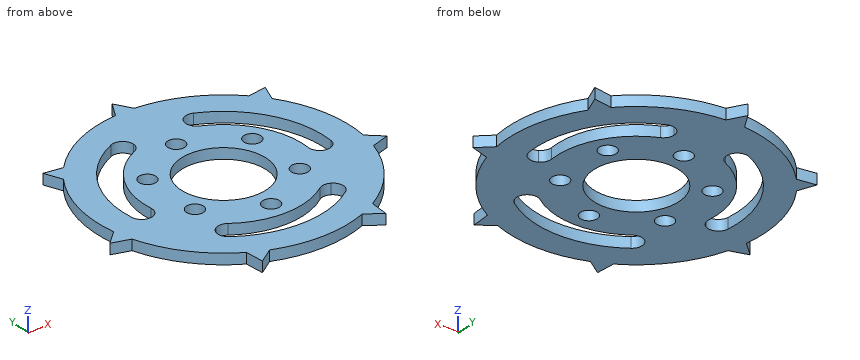
Autodesk Fusion 360 part; units mm, degrees
sketch "Sketch1" plane through (0, 0, 0) normal (0, 0, 1) x (1, 0, 0)
  circle A0 centre (0, 0) radius 24
  circle A1 centre (0, 0) radius 11.5
  line L0 (0, 0) -> (0, 11.5)
  line L1 (0, 0) -> (-9.9593, 5.75)
  line L2 (0, 0) -> (9.9593, 5.75)
  line L3 (0, 0) -> (9.9593, -5.75)
  line L4 (0, 0) -> (0, -11.5)
  line L5 (0, 0) -> (-9.9593, -5.75)
  circle A2 centre (0, 11.5) radius 1.6
  circle A3 centre (9.9593, 5.75) radius 1.6
  circle A4 centre (9.9593, -5.75) radius 1.6
  circle A5 centre (0, -11.5) radius 1.6
  circle A6 centre (-9.9593, -5.75) radius 1.6
  circle A7 centre (-9.9593, 5.75) radius 1.6
  line L6 (0, 11.5) -> (-5, 11.5)
  line L7 (0, 11.5) -> (5, 11.5)
  line L8 (9.9593, -5.75) -> (7.4593, -10.0801)
  line L9 (9.9593, -5.75) -> (12.4593, -1.4199)
  line L10 (-9.9593, -5.75) -> (-7.4593, -10.0801)
  line L11 (-9.9593, -5.75) -> (-12.4593, -1.4199)
  circle A8 centre (0, 0) radius 19
  line L12 (-5, 11.5) -> (-5, 10.3562)
  line L13 (5, 11.5) -> (5, 10.3562)
  line L14 (12.4593, -1.4199) -> (11.4687, -0.848)
  line L15 (7.4593, -10.0801) -> (6.4687, -9.5082)
  line L16 (-7.4593, -10.0801) -> (-6.4687, -9.5082)
  line L17 (-12.4593, -1.4199) -> (-11.4687, -0.848)
  line L18 (-12.4593, -1.4199) -> (-18.3745, -4.835)
  line L19 (-7.4593, -10.0801) -> (-13.3745, -13.4953)
  line L20 (7.4593, -10.0801) -> (13.3745, -13.4953)
  line L21 (12.4593, -1.4199) -> (18.3745, -4.835)
  line L22 (5, 11.5) -> (5, 18.3303)
  line L23 (-5, 11.5) -> (-5, 18.3303)
  circle A9 centre (0, 0) radius 8
  circle A10 centre (0, 0) radius 15
  line L24 (0, 24) -> (-15.4269, 18.3851)
  line L25 (-15.4269, 18.3851) -> (-23.6354, 4.1676)
  line L26 (-23.6354, 4.1676) -> (-20.7846, -12)
  line L27 (-20.7846, -12) -> (-8.2085, -22.5526)
  line L28 (-8.2085, -22.5526) -> (8.2085, -22.5526)
  line L29 (8.2085, -22.5526) -> (20.7846, -12)
  line L30 (20.7846, -12) -> (23.6354, 4.1676)
  line L31 (23.6354, 4.1676) -> (15.4269, 18.3851)
  line L32 (15.4269, 18.3851) -> (0, 24)
  line L33 (0, 24) -> (0.2615, 26.9886)
  line L34 (0, 24) -> (3, 24) construction
  line L35 (0.2615, 26.9886) -> (-1.883, 23.926)
  line L36 (0.2615, 26.9886) -> (4.0002, 26.9886) construction
  dimension "d1" = 48
  dimension "d2" = 23
  dimension "d3" = 3.2
  dimension "d4" = 3.2
  dimension "d5" = 3.2
  dimension "d6" = 3.2
  dimension "d7" = 3.2
  dimension "d8" = 3.2
  dimension "d9" = 5
  dimension "d10" = 5
  dimension "d11" = 5
  dimension "d12" = 5
  dimension "d13" = 5
  dimension "d14" = 38
  dimension "d15" = 16
  dimension "d16" = 30
  dimension "d17" = 85
  dimension "d18" = 3
  dimension "d19" = 125
extrude "Extrude1" add sketch "Sketch1" along normal blind 2 contours A0 L30 | A0 L31 | L24 L25 L26 L27 L28 L29 L30 L31 L32 | A0 L29 | A0 L32 | A0 L28 | A0 L24 | A0 L27 | A0 L25 | A0 L26 | A1 L2 L3 A3 A4 A9 | A1 A4 L9 L14 | A1 A3 L13 L14 L21 L22 A10 | A4 L8 L9 L20 L21 A10 | A1 L3 L4 A4 A5 A9 | A8 L20 L21 A10 | A1 L0 L2 A2 A3 A9 | A1 A4 L8 L15 | A1 A5 L15 L16 L19 L20 A10 | A1 L4 L5 A5 A6 A9 | A6 L10 L11 L18 L19 A10 | A8 L18 L19 A10 | A8 L22 L23 A10 | A2 L6 L7 L22 L23 A10 | A1 A2 L7 L13 | A1 L0 L1 A2 A7 A9 | A1 L1 L5 A6 A7 A9 | A1 A6 L10 L16 | A1 A7 L12 L17 L18 L23 A10 | A1 A6 L11 L17 | A1 A2 L6 L12
fillet "Fillet1" radius 2 12 edges at (5, 18.3303, 1) (5, 14.1421, 1) (14.7474, -2.7409, 1) (18.3745, -4.835, 1) (13.3745, -13.4953, 1) (9.7474, -11.4012, 1) (-9.7474, -11.4012, 1) (-13.3745, -13.4953, 1) (-18.3745, -4.835, 1) (-14.7474, -2.7409, 1) (-5, 14.1421, 1) (-5, 18.3303, 1)
sketch "Sketch2" plane through (0, 0, 2) normal (0, 0, 1) x (-1, 0, 0)
  circle A0 centre (9.9593, 5.75) radius 1.6
  circle A1 centre (0, 0) radius 8
  circle A2 centre (0, -11.5) radius 1.6
  arc A3 (8.7498, 12.1837) -> (11.083, 15.4326) centre (9.9164, 13.8081) ccw
  arc A4 (8.7498, 12.1837) -> (-8.7498, 12.1837) centre (0, 0) ccw
  arc A5 (-11.083, 15.4326) -> (-8.7498, 12.1837) centre (-9.9164, 13.8081) ccw
  arc A6 (11.083, 15.4326) -> (-11.083, 15.4326) centre (0, 0) ccw
  circle A7 centre (9.9593, -5.75) radius 1.6
  arc A8 (6.1765, -13.6694) -> (7.8235, -17.3145) centre (7, -15.4919) ccw
  arc A9 (6.1765, -13.6694) -> (14.9262, 1.4857) centre (0, 0) ccw
  arc A10 (18.9066, 1.8819) -> (14.9262, 1.4857) centre (16.9164, 1.6838) ccw
  arc A11 (7.8235, -17.3145) -> (18.9066, 1.8819) centre (0, 0) ccw
  arc A12 (-18.9066, 1.8819) -> (-7.8235, -17.3145) centre (0, 0) ccw
  arc A13 (-14.9262, 1.4857) -> (-18.9066, 1.8819) centre (-16.9164, 1.6838) ccw
  arc A14 (-14.9262, 1.4857) -> (-6.1765, -13.6694) centre (0, 0) ccw
  arc A15 (-7.8235, -17.3145) -> (-6.1765, -13.6694) centre (-7, -15.4919) ccw
  circle A16 centre (-9.9593, -5.75) radius 1.6
  circle A17 centre (0, 11.5) radius 1.6
  circle A18 centre (-9.9593, 5.75) radius 1.6
  circle A19 centre (0, 0) radius 24
  line L0 (0, -8) -> (0, -13.1)
  line L1 (0, -24) -> (3.0935, -24) construction
  line L2 (0, -24) -> (0, -27)
  line L3 (0, -24) -> (3.0102, -24) construction
  line L4 (0, -27) -> (1.7698, -23.9347)
  line L5 (0, -27) -> (-1.7698, -23.9347)
  arc A20 (0, -27) -> (0, -27) centre (0, 0) ccw
  arc A21 (-1.7698, -23.9347) -> (1.7698, -23.9347) centre (0, 0) ccw
  line L6 (21.1095, -16.8342) -> (19.8163, -13.5393)
  line L7 (21.1095, -16.8342) -> (17.6094, -16.3067)
  arc A22 (17.6094, -16.3067) -> (19.8163, -13.5393) centre (0, 0) ccw
  line L8 (26.3231, 6.0081) -> (22.9408, 7.0514)
  line L9 (26.3231, 6.0081) -> (23.7284, 3.6006)
  arc A23 (23.7284, 3.6006) -> (22.9408, 7.0514) centre (0, 0) ccw
  line L10 (11.7149, 24.3262) -> (8.7903, 22.3323)
  line L11 (11.7149, 24.3262) -> (11.9794, 20.7965)
  arc A24 (11.9794, 20.7965) -> (8.7903, 22.3323) centre (0, 0) ccw
  line L12 (-11.7149, 24.3262) -> (-11.9794, 20.7965)
  line L13 (-11.7149, 24.3262) -> (-8.7903, 22.3323)
  arc A25 (-8.7903, 22.3323) -> (-11.9794, 20.7965) centre (0, 0) ccw
  line L14 (-26.3231, 6.0081) -> (-23.7284, 3.6006)
  line L15 (-26.3231, 6.0081) -> (-22.9408, 7.0514)
  arc A26 (-22.9408, 7.0514) -> (-23.7284, 3.6006) centre (0, 0) ccw
  line L16 (-21.1095, -16.8342) -> (-17.6094, -16.3067)
  line L17 (-21.1095, -16.8342) -> (-19.8163, -13.5393)
  arc A27 (-19.8163, -13.5393) -> (-17.6094, -16.3067) centre (0, 0) ccw
  dimension "d24" = 54
  dimension "d30" = 30
  dimension "d46" = 360
extrude "Extrude5" add sketch "Sketch2" against normal blind 2 contours A19 L8 L9 A23 | A19 L6 L7 A22 | A19 L10 L11 A24 | A19 L2 L4 A21 | A19 L2 L5 A21 | A19 L12 L13 A25 | A19 L16 L17 A27 | A19 L14 L15 A26
Build history of the part. All positions in model axes, mm. Round coordinates to 2 decimals unless told otherwise and drop trailing zeros. Loops run counter-clockwise (first coordinate to the right, second up) from the corner with the lowest first, then second, coordinate; pieces in that order, holes last. Notation, with made-up numbers: M 11,-36.75 L 62,-36.75 A25 ccw 62,-4.75 Z; hole C -34.75,14 d8. An arc over 180 degrees is marked long. Answer as CSV lines item,"result".
1. Wall check: probe 1 along X at (y, z) = (0, 1.2); probe 2 along X at (y, z) = (3, 1.75); probe 3 along Y at (x, z) = (-10, 0.2). Give the ranges that are in metal, low to high. Write a range as [from, to].
Resolved:
probe 1,"x = [-24, -19], [-15, -8], [8, 15], [19, 24]"
probe 2,"x = [-23.81, -18.76], [-14.7, -7.42], [7.42, 14.7], [18.76, 23.81]"
probe 3,"y = [-23.16, -16.16], [-11.81, -7.35], [-4.15, 4.15], [7.35, 11.18], [16.16, 21.82]"
2. Flat gauge pins, fed straight in: P1, Ø1, axis at y = 18, z = 0.5, coming from the -X side; P2, Ø5, axis at x = 9.96, y = 5.75, coming from the -Z side. Where does each tip first touch, or does it go through?
Resolved:
P1,"stops at x = -16.42"
P2,"stops at z = 0"
3. Cut at C-C on y = 5.75. Write the cut outline in (x, z).
Resolved:
outline,"M -23.3,0 L -18.11,0 L -18.11,2 L -23.3,2 Z; M -13.85,0 L -11.56,0 L -11.56,2 L -13.85,2 Z; M -8.36,0 L -5.56,0 L -5.56,2 L -8.36,2 Z; M 5.56,0 L 8.36,0 L 8.36,2 L 5.56,2 Z; M 11.56,0 L 13.85,0 L 13.85,2 L 11.56,2 Z; M 18.11,0 L 23.3,0 L 23.3,2 L 18.11,2 Z"
4. Cut at A-A on y = 0. Write the cut outline in (x, z).
Resolved:
outline,"M -24,0 L -19,0 L -19,2 L -24,2 Z; M -15,0 L -8,0 L -8,2 L -15,2 Z; M 8,0 L 15,0 L 15,2 L 8,2 Z; M 19,0 L 24,0 L 24,2 L 19,2 Z"
5. Cut at D-D on x = -22. Write the cut outline in (y, z), then the cut area to 3 significant figures.
Resolved:
outline,"M -9.59,0 L 9.59,0 L 9.59,2 L -9.59,2 Z"
area,"38.4 mm²"
6. Cut at B-B on y = -14. Write the cut outline in (x, z), then the cut area to 3 significant figures.
Resolved:
outline,"M -19.49,0 L -11.91,0 L -11.91,2 L -19.49,2 Z; M -5.39,0 L 5.39,0 L 5.39,2 L -5.39,2 Z; M 11.91,0 L 19.49,0 L 19.49,2 L 11.91,2 Z"
area,"51.9 mm²"
